Here's how the part is built. I have some questions about the finished solid (model axes, mm). A direction names the side the tool comes from. Give positions to 0.01 mm unless a question says otherwise; leave off trailing zeros. Loops run counter-clockwise (first coordinate to the right, second up) from the corner with the lowest first, then second, coordinate; pieces in that order, holes last.
Q1. Will these pins go through, and if not, where does the flat tip stop? P1, Ø17, axis at x = 37, z = 16, coming from the -Y side; P2, Ø5, axis at x = -6, z = -29, coming from the -Y side; P3, Ø4, axis at y = 76, z = 13, coming from the +X side.
Q2. If we section it at A-A (z = 0): Please give me the cut outline in (x, y), plus the area to 3 significant figures.
Q3. I need wall thicknesses on line 1 (X direction, y = 37.5, z = 31.5); line 2 (X direction, y = 27.5, z = -10.5); line 3 (X direction, y = 90, z = -35). Which ranges of each line are inside material? Lowest first, please.
Q4. For faces 4 (the face through (-2.73, 57.89, 47.15)), 5 (the face through (37.32, -4.93, -1.63)), 6 (the face through (29.901, 31.516, 0.56)), 7 (the face through (-2.73, 57.89, -47.15)), which set-ups out of +Z, -Z, +X, -X, +Y, -Y let a thin tool reach every point of the face, with its end or its side?
Q5. We'd pull the mould along X, two halves only. Please class faces 1 (the face through (67.67, 4.93, 0.7)), 2 (the face through (30.261, 28.366, 47.148)), 3 (the face through (30, -10, 0)): +X half, -X half, draft (parallel to the pull), parting line (faces both ways), or undercut.
from build123d import *

# Parameters (mm, degrees)
BOSS_EXTRUDE1_DEPTH = 50
SKETCH4_R           = 7.5
BOSS_EXTRUDE2_DEPTH = 10
FILLET1_R           = 10
CHAMFER1_SIZE       = 2


with BuildPart() as part:
    # Sketch3 → Boss-Extrude1 (new, symmetric)
    with BuildSketch(Plane.XY):
        with BuildLine():
            Line((-50.714191409, 108.756934444), (0, 0))
            Line((0, 0), (57.1, 0))
            Line((57.1, 0), (78.545069205, 10))
            Line((78.545069205, 10), (70.068082541, 28.178956567))
            ThreePointArc((70.068082541, 28.178956567), (58.782329667, 38.520443748), (43.489561565, 37.852747073))
            Line((43.489561565, 37.852747073), (15.92675652, 25))
            Line((15.92675652, 25), (-19.604131498, 101.196235247))
            ThreePointArc((-19.604131498, 101.196235247), (-30.889884372, 111.537722428), (-46.182652474, 110.870025753))
            Line((-46.182652474, 110.870025753), (-50.714191409, 108.756934444))
        make_face()
    extrude(amount=BOSS_EXTRUDE1_DEPTH, both=True)

    # Sketch4 → Boss-Extrude2 (add)
    with BuildSketch(Plane.XZ):
        with Locations(Location((30, 0, 0), (0, 0, 90))):
            Circle(SKETCH4_R)
    extrude(amount=BOSS_EXTRUDE2_DEPTH)

    # Fillet1
    fillet1_edges = [part.edges().sort_by_distance(p)[0] for p in [
        (29.708159043, 31.426373536, -50),
        (58.782329667, 38.520443748, -50),
        (74.306575873, 19.089478283, -50),
        (-48.448421941, 109.813480099, -50),
        (74.306575873, 19.089478283, 50),
        (58.782329667, 38.520443748, 50),
        (29.708159043, 31.426373536, 50),
        (-1.838687489, 63.098117624, 50),
        (-30.889884372, 111.537722428, 50),
        (-48.448421941, 109.813480099, 50),
        (-30.889884372, 111.537722428, -50),
        (-1.838687489, 63.098117624, -50),
    ]]
    fillet(fillet1_edges, radius=FILLET1_R)

    # Chamfer1
    chamfer1_edges = [part.edges().sort_by_distance(p)[0] for p in [
        (-23.244004396, 49.846928287, -50),
        (-23.244004396, 49.846928287, 50),
        (-50.714191409, 108.756934444, 0),
        (-49.476371179, 106.102420395, 47.071067812),
        (-49.476371179, 106.102420395, -47.071067812),
    ]]
    chamfer(chamfer1_edges, length=CHAMFER1_SIZE)


solid = part.part
Check sheet entries:
1. P1: stops at y = 0
1. P2: stops at y = 7.51
1. P3: stops at x = -6.92
2. outline: (-49.87, 106.94) - (0, 0) - (22.5, 0) - (22.5, -10) - (37.5, -10) - (37.5, 0) - (57.1, 0) - (78.55, 10) - (70.07, 28.18) arc R20 ccw to (43.49, 37.85) - (15.93, 25) - (-19.6, 101.2) arc R20 ccw to (-46.18, 110.87) - (-48.9, 109.6) - close
2. area: 4,970 mm2
3. line 1: x = -17.49 to 10.1, 42.73 to 61.11
3. line 2: x = -12.82 to 14.76, 21.29 to 70.38
3. line 3: x = -41.97 to -14.38
4. face 4: +Z, +Y
4. face 5: -Y
4. face 6: +Z, -Z, +Y
4. face 7: -Z, +Y
5. face 1: +X half
5. face 2: undercut
5. face 3: draft
